Source: three-view drawing plus pictorial views. Frame: mm from the lowest corner of the part. A direction names the side the tool comes from. Round coordinates to 2 decimals unless told otherwise and drop trailing zeros. Loops run counter-clockwise (first coordinate to the right, second up) from the corner with the lowest first, then second, coordinate; pieces in that order, holes last. Notation, with made-up numbers: M 56,80 L 106,80 A21 ccw 106,116 Z; hole C 21,16 d1. An arc over 180 degrees is marked long. Return JSON: item names as keys, results as strings. Group by question number.
1) Access query for the marked faces 1 and 2. Directions: +Z, -Z, +X, -X, +Y, -Y. A direction counts if a zero-diameter tool reaches every point of the face in a straight line with its end or side. Return the directions, or none.
2) Section C-C (z = 62). Output: boundary loops of the cut face in (x, y), plus the area to 3 significant figures.
3) Section B-B (x = 12.7). Output: boundary loops of the cut face in (y, z).
4) Section D-D (y = 23.75). Output: boundary loops of the cut face in (x, z).
5) Material intervals for line 1 (Z direction, x = 6.75, y = 10); line 2 (Y direction, x = 12.75, z = 17); line 3 (Y direction, x = 5.5, z = 53), sorted ascending. Write a range as from..to.
6) Contact query for flat-ended pins moving along their axis: P1, Ø6, axis at y = 23, z = 37, coming from the +X side; P2, Ø12, axis at y = 18.5, z = 73, coming from the +X side; P3, Ø4, axis at y = 7.5, z = 77.5, coming from the -X side; P4, Ø1, axis at x = 7.5, z = 11, coming from the -Y side. Output: stop coordinate, or through.
7) Section A-A (y = 12.7). Output: boundary loops of the cut face in (x, z), plus the area to 3 significant figures.
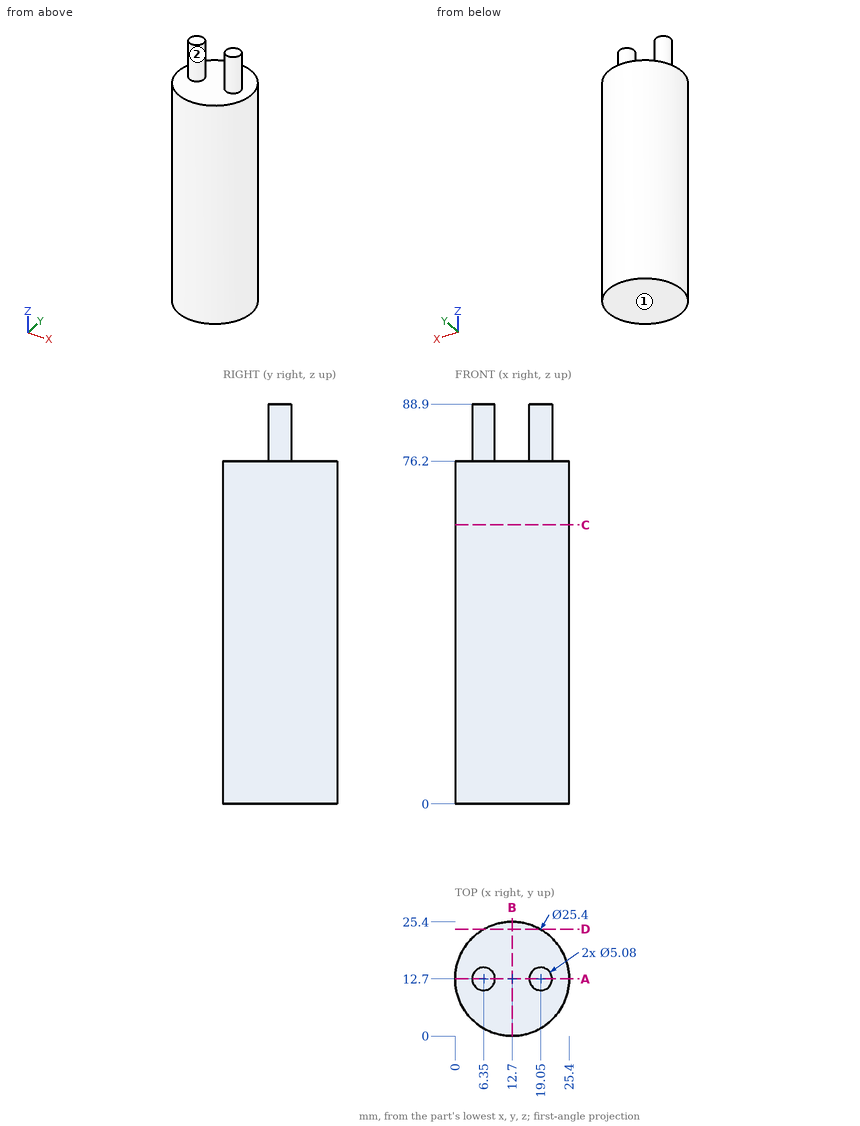
Returned:
{
 "1": {"face 1": "-Z, +X, -X, +Y, -Y", "face 2": "+Z"},
 "2": {"outline": "C 12.7,12.7 d25.4", "area": "507 mm^2"},
 "3": {"outline": "M 0,0 L 25.4,0 L 25.4,76.2 L 0,76.2 Z"},
 "4": {"outline": "M 6.44,0 L 18.96,0 L 18.96,76.2 L 6.44,76.2 Z"},
 "5": {"line 1": "z = 0..76.2", "line 2": "y = 0..25.4", "line 3": "y = 2.24..23.16"},
 "6": {"P1": "stops at x = 23.09", "P2": "stops at x = 25.4", "P3": "stops at x = 0.54", "P4": "stops at y = 0.9"},
 "7": {"outline": "M 0,0 L 25.4,0 L 25.4,76.2 L 21.59,76.2 L 21.59,88.9 L 16.51,88.9 L 16.51,76.2 L 8.89,76.2 L 8.89,88.9 L 3.81,88.9 L 3.81,76.2 L 0,76.2 Z", "area": "2,060 mm^2"}
}
